from build123d import *

# Parameters (mm, degrees)
BOSS_EXTRUDE1_DEPTH     = 609.6
CUT_EXTRUDE1_DEPTH      = 254
CUT_EXTRUDE1_DEPTH_BACK = 254
SKETCH2_R               = 1.75
SKETCH4_R               = 1.75
CUT_EXTRUDE2_DEPTH      = 254
SKETCH6_W               = 6.35
SKETCH6_H               = 6.35
CUT_EXTRUDE4_DEPTH      = 90.678
SKETCH7_W               = 6.35
SKETCH7_H               = 6.35
CUT_EXTRUDE5_DEPTH      = 122.174
SKETCH8_W               = 63.5
SKETCH8_H               = 228.6
BOSS_EXTRUDE2_DEPTH     = 3.33375
SKETCH9_R               = 2.75
CUT_EXTRUDE6_DEPTH      = 100.584
SKETCH11_W              = 12.7
SKETCH11_H              = 12.7
CUT_EXTRUDE8_DEPTH      = 31.496


with BuildPart() as part:
    # Sketch1 → Boss-Extrude1 (new body)
    with BuildSketch(Plane(origin=(0, 0, 0), x_dir=(0, 1, 0), z_dir=(0, 0, 1))):
        Polygon((28.41625, 28.41625), (28.41625, -28.41625), (6.985, -28.41625), (6.985, -31.75), (31.75, -31.75), (31.75, 31.75), (-31.75, 31.75), (-31.75, -31.75), (-6.985, -31.75), (-6.985, -28.41625), (-28.41625, -28.41625), (-28.41625, 28.41625), align=None)
    extrude(amount=BOSS_EXTRUDE1_DEPTH)

    # Sketch2 → Cut-Extrude1 (cut, two sides: drawn at the far end of the back side and taken through both)
    with BuildSketch(Plane(origin=(0, 0, 0), x_dir=(-1, 0, 0), z_dir=(0, 1, 0)).offset(-CUT_EXTRUDE1_DEPTH_BACK)):
        with Locations(Location((-24.05, 15.875, 0), (0, 0, 270))):
            Circle(SKETCH2_R)
        with Locations(Location((24.05, 15.875, 0), (0, 0, 270))):
            Circle(SKETCH2_R)
    extrude(amount=CUT_EXTRUDE1_DEPTH + CUT_EXTRUDE1_DEPTH_BACK, mode=Mode.SUBTRACT)

    # Sketch4 → Cut-Extrude2 (cut)
    with BuildSketch(Plane.YZ.offset(31.75)):
        with Locations((24.05, 28.575)):
            Circle(SKETCH4_R)
        with Locations((-24.05, 28.575)):
            Circle(SKETCH4_R)
    extrude(amount=-CUT_EXTRUDE2_DEPTH, mode=Mode.SUBTRACT)

    # Sketch6 → Cut-Extrude4 (cut)
    with BuildSketch(Plane.YZ.offset(31.75)):
        with Locations((17.05, 15.875)):
            Rectangle(SKETCH6_W, SKETCH6_H)
        with Locations((-17.05, 15.875)):
            Rectangle(SKETCH6_W, SKETCH6_H)
    extrude(amount=-CUT_EXTRUDE4_DEPTH, mode=Mode.SUBTRACT)

    # Sketch7 → Cut-Extrude5 (cut)
    with BuildSketch(Plane(origin=(0, 31.75, 0), x_dir=(-1, 0, 0), z_dir=(0, 1, 0))):
        with Locations((-17.05, 28.575)):
            Rectangle(SKETCH7_W, SKETCH7_H)
        with Locations((17.05, 28.575)):
            Rectangle(SKETCH7_W, SKETCH7_H)
    extrude(amount=-CUT_EXTRUDE5_DEPTH, mode=Mode.SUBTRACT)

    # Sketch8 → Boss-Extrude2 (add)
    with BuildSketch(Plane.YZ.offset(31.75)):
        with Locations((0, 495.3)):
            Rectangle(SKETCH8_W, SKETCH8_H)
    extrude(amount=-BOSS_EXTRUDE2_DEPTH)

    # Sketch9 → Cut-Extrude6 (cut)
    with BuildSketch(Plane.YZ.offset(31.75)):
        with Locations((-16.812006, 599.52001)):
            Circle(SKETCH9_R)
        with Locations((-16.812006, 543.47999)):
            Circle(SKETCH9_R)
        with Locations((16.812006, 543.47999)):
            Circle(SKETCH9_R)
        with Locations((16.812006, 599.52001)):
            Circle(SKETCH9_R)
    extrude(amount=-CUT_EXTRUDE6_DEPTH, mode=Mode.SUBTRACT)

    # Sketch11 → Cut-Extrude8 (cut)
    with BuildSketch(Plane(origin=(0, -28.41625, 0), x_dir=(-1, 0, 0), z_dir=(0, 1, 0))):
        with Locations((0, 603.25)):
            Rectangle(SKETCH11_W, SKETCH11_H)
    extrude(amount=-CUT_EXTRUDE8_DEPTH, mode=Mode.SUBTRACT)


solid = part.part
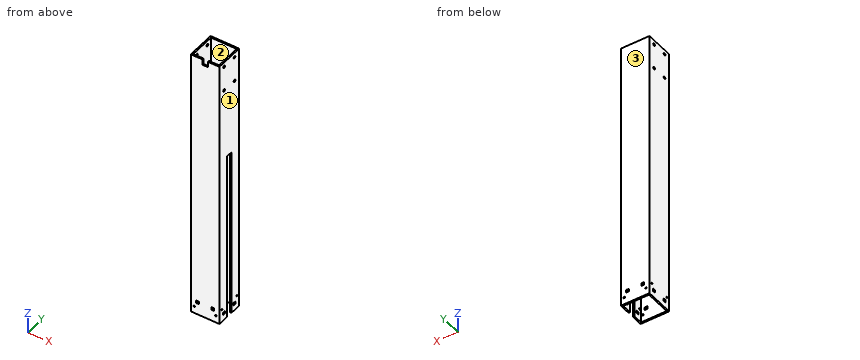
Here's how the part is built. I have some questions about the finished solid (model axes, mm). Face numbers are marked on the shaded views. Round coordinates to 2 decimals unless told otherwise and drop trailing zeros. Order: outer loops, then holes, each group sorted by start corner. A loop starts at its lowest first (then second) coordinate and runs counter-clockwise, first axis right, second up. Notation, with made-up numbers: M 65.5,-34 L 119.5,-34 A16 ccw 119.5,-5 Z; hole C 44,51 d1. An arc over 180 degrees is marked long. Return JSON: item names as keys, results as strings. Group by question number.
1. If we mould it in two halves opening along Y, with no side actions, what happens to the marked faces 1, 2 and 3? For each: pulls with the +Y half, pulls with the -Y half, needs draft (parallel to the pull), parting line crosses it, or undercut.
2. Please list where these lines run through material, in increasing order: probe 1 along Y at (x, z) = (-6, 116.5); probe 2 along Z at (x, y) = (15, 28.5).
3. I'm going to push flat-ended pins straight in: pin 1 Ø12 at (x, y) = (-24, -4.5) entering from +Z; pin 2 Ø3 at (x, z) = (24.05, 15.875) entering from +Y. Where does each tip first touch, or does it pass through?
4. If we section it at B-B on z = 195.5: List the corners of the cut face in (x, y) for me (3 decimals), then the cut area to 3 significant figures.
5. If we section it at A-A on z = 454.5: List the corners of the cut face in (x, y) for me, then the cut area to 3 significant figures.
Reply:
{
 "1": {"face 1": "needs draft", "face 2": "undercut", "face 3": "pulls with the +Y half"},
 "2": {"probe 1": "-31.75 to -28.42, 28.42 to 31.75", "probe 2": "0 to 25.4, 31.75 to 609.6"},
 "3": {"pin 1": "z = 609.6", "pin 2": "through"},
 "4": {"outline": "M -31.75,-31.75 L 31.75,-31.75 L 31.75,-6.985 L 28.416,-6.985 L 28.416,-28.416 L -28.416,-28.416 L -28.416,28.416 L 28.416,28.416 L 28.416,6.985 L 31.75,6.985 L 31.75,31.75 L -31.75,31.75 Z", "area": "756 mm^2"},
 "5": {"outline": "M -31.75,-31.75 L 31.75,-31.75 L 31.75,31.75 L -31.75,31.75 Z; hole M -28.42,-28.42 L 28.42,-28.42 L 28.42,28.42 L -28.42,28.42 Z", "area": "802 mm^2"}
}
